Work out the finished part from the listing and answer in its coordinate system (mm). Face numbers are marked on the shaded views. A direction names the side the tool comes from. Round coordinates to 2 decimals unless told otherwise and drop trailing zeros. Order: outer loops, then holes, each group sorted by start corner. A loop starts at its lowest first (then second) coordinate and runs counter-clockwise, first axis right, second up. Notation, with made-up numbers: (-35, -21.5) - (23, -21.5) arc R14 cw to (23, -11.5) - close; hole circle Ø2 at (59, 7.5). An arc over 180 degrees is marked (long way). Answer in a Markdown table with one row per item.
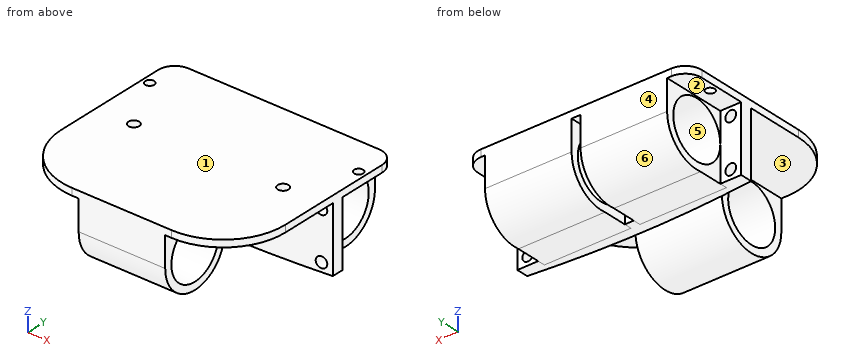
from build123d import *

# Parameters (mm, degrees)
SKETCH1_R            = 1.79994
SKETCH1_R_2          = 1.5
BOSS_EXTRUDE1_DEPTH  = 7
SKETCH2_W            = 75
SKETCH2_H            = 13.099999962
SKETCH2_R            = 2.6999438
SKETCH2_R_2          = 2.499995
SKETCH2_R_3          = 1.3498449
BOSS_EXTRUDE2_DEPTH  = 6.987999994
SKETCH2_3_R          = 2.6999438
SKETCH2_3_R_2        = 1.3498449
CUT_EXTRUDE1_DEPTH   = 2.5
SKETCH5_W            = 75
SKETCH5_H            = 13.099999962
CUT_EXTRUDE3_DEPTH   = 21.082
SKETCH6_W            = 75
SKETCH6_H            = 7
BOSS_EXTRUDE3_DEPTH  = 9.5
SKETCH8_W            = 75
SKETCH8_H            = 38.030205227
CUT_EXTRUDE4_DEPTH   = 4.666
SKETCH10_W           = 75
SKETCH10_H           = 2.334
BOSS_EXTRUDE5_DEPTH  = 35
SKETCH11_R           = 1.79994
CUT_EXTRUDE5_DEPTH   = 5
SKETCH15_W           = 44.653530321
SKETCH15_H           = 13.617301916
SKETCH15_W_2         = 11.728266088
SKETCH15_H_2         = 5.987537529
BOSS_EXTRUDE7_DEPTH  = 2.334
SKETCH16_R           = 9.5
BOSS_EXTRUDE9_DEPTH  = 29
SKETCH17_R           = 9.5
BOSS_EXTRUDE11_DEPTH = 14.5
FILLET5_R            = 20.828
FILLET6_R            = 5.588
BOSS_EXTRUDE13_DEPTH = 21.905881
CUT_EXTRUDE6_REACH   = 46
SKETCH21_R           = 1.8


with BuildPart() as part:
    # Sketch1 → Boss-Extrude1 (new body)
    with BuildSketch(Plane.XY):
        with BuildLine():
            Line((37.5, -10.5), (30, -10.5))
            ThreePointArc((30, -10.5), (25, -15.5), (20, -10.5))
            Line((20, -10.5), (5, -10.5))
            ThreePointArc((5, -10.5), (0, -15.5), (-5, -10.5))
            Line((-5, -10.5), (-20, -10.5))
            ThreePointArc((-20, -10.5), (-25, -15.5), (-30, -10.5))
            Line((-30, -10.5), (-37.5, -10.5))
            Line((-37.5, -10.5), (-37.5, 10.5))
            Line((-37.5, 10.5), (37.5, 10.5))
            Line((37.5, 10.5), (37.5, -10.5))
        make_face()
        with Locations((-25, -10.5)):
            Circle(SKETCH1_R, mode=Mode.SUBTRACT)
        with Locations((0, -10.5)):
            Circle(SKETCH1_R, mode=Mode.SUBTRACT)
        with Locations((25, -10.5)):
            Circle(SKETCH1_R, mode=Mode.SUBTRACT)
        with Locations((-35, 8)):
            Circle(SKETCH1_R_2, mode=Mode.SUBTRACT)
        with Locations((-15, 8)):
            Circle(SKETCH1_R_2, mode=Mode.SUBTRACT)
        with Locations((-10, 8)):
            Circle(SKETCH1_R_2, mode=Mode.SUBTRACT)
        with Locations((10, 8)):
            Circle(SKETCH1_R_2, mode=Mode.SUBTRACT)
        with Locations((35, 8)):
            Circle(SKETCH1_R_2, mode=Mode.SUBTRACT)
        with Locations((15, 8)):
            Circle(SKETCH1_R_2, mode=Mode.SUBTRACT)
    extrude(amount=BOSS_EXTRUDE1_DEPTH)

    # Sketch2 → Boss-Extrude2 (add)
    with BuildSketch(Plane(origin=(0, 2.24999999, 0), x_dir=(1, 0, 0), z_dir=(0, 1, 0))):
        with Locations((0, -13.549999981)):
            Rectangle(SKETCH2_W, SKETCH2_H)
        with Locations((31.0001404, -13.549999981)):
            Circle(SKETCH2_R, mode=Mode.SUBTRACT)
        with Locations((-31.0001404, -13.549999981)):
            Circle(SKETCH2_R, mode=Mode.SUBTRACT)
        with Locations((-25, -13.549999981)):
            Circle(SKETCH2_R_2, mode=Mode.SUBTRACT)
        with Locations((-6.0001404, -13.549999981)):
            Circle(SKETCH2_R, mode=Mode.SUBTRACT)
        with Locations((6.0001404, -13.549999981)):
            Circle(SKETCH2_R, mode=Mode.SUBTRACT)
        with Locations((0, -13.549999981)):
            Circle(SKETCH2_R_2, mode=Mode.SUBTRACT)
        with Locations((-18.9998596, -13.549999981)):
            Circle(SKETCH2_R, mode=Mode.SUBTRACT)
        with Locations((25, -13.549999981)):
            Circle(SKETCH2_R_2, mode=Mode.SUBTRACT)
        with Locations((18.9998596, -13.549999981)):
            Circle(SKETCH2_R, mode=Mode.SUBTRACT)
        with Locations((-31.0001404, -13.549999981)):
            Circle(SKETCH2_R)
        with Locations((-31.0001404, -13.549999981)):
            Circle(SKETCH2_R_3, mode=Mode.SUBTRACT)
        with Locations((-18.9998596, -13.549999981)):
            Circle(SKETCH2_R)
        with Locations((-18.9998596, -13.549999981)):
            Circle(SKETCH2_R_3, mode=Mode.SUBTRACT)
        with Locations((-6.0001404, -13.549999981)):
            Circle(SKETCH2_R)
        with Locations((-6.0001404, -13.549999981)):
            Circle(SKETCH2_R_3, mode=Mode.SUBTRACT)
        with Locations((6.0001404, -13.549999981)):
            Circle(SKETCH2_R)
        with Locations((6.0001404, -13.549999981)):
            Circle(SKETCH2_R_3, mode=Mode.SUBTRACT)
        with Locations((18.9998596, -13.549999981)):
            Circle(SKETCH2_R)
        with Locations((18.9998596, -13.549999981)):
            Circle(SKETCH2_R_3, mode=Mode.SUBTRACT)
        with Locations((31.0001404, -13.549999981)):
            Circle(SKETCH2_R)
        with Locations((31.0001404, -13.549999981)):
            Circle(SKETCH2_R_3, mode=Mode.SUBTRACT)
    extrude(amount=-BOSS_EXTRUDE2_DEPTH)

    # Sketch2<3> → Cut-Extrude1 (cut)
    with BuildSketch(Plane(origin=(0, 2.24999999, 0), x_dir=(1, 0, 0), z_dir=(0, 1, 0))):
        with Locations((-31.0001404, -13.549999981)):
            Circle(SKETCH2_3_R)
        with Locations((-31.0001404, -13.549999981)):
            Circle(SKETCH2_3_R_2, mode=Mode.SUBTRACT)
        with Locations((-18.9998596, -13.549999981)):
            Circle(SKETCH2_3_R)
        with Locations((-18.9998596, -13.549999981)):
            Circle(SKETCH2_3_R_2, mode=Mode.SUBTRACT)
        with Locations((-6.0001404, -13.549999981)):
            Circle(SKETCH2_3_R)
        with Locations((-6.0001404, -13.549999981)):
            Circle(SKETCH2_3_R_2, mode=Mode.SUBTRACT)
        with Locations((6.0001404, -13.549999981)):
            Circle(SKETCH2_3_R)
        with Locations((6.0001404, -13.549999981)):
            Circle(SKETCH2_3_R_2, mode=Mode.SUBTRACT)
        with Locations((18.9998596, -13.549999981)):
            Circle(SKETCH2_3_R)
        with Locations((18.9998596, -13.549999981)):
            Circle(SKETCH2_3_R_2, mode=Mode.SUBTRACT)
        with Locations((31.0001404, -13.549999981)):
            Circle(SKETCH2_3_R)
        with Locations((31.0001404, -13.549999981)):
            Circle(SKETCH2_3_R_2, mode=Mode.SUBTRACT)
    extrude(amount=-CUT_EXTRUDE1_DEPTH, mode=Mode.SUBTRACT)

    # Sketch5 → Cut-Extrude3 (cut)
    with BuildSketch(Plane(origin=(0, 2.24999999, 0), x_dir=(1, 0, 0), z_dir=(0, 1, 0))):
        with Locations((0, -13.549999981)):
            Rectangle(SKETCH5_W, SKETCH5_H)
    extrude(amount=-CUT_EXTRUDE3_DEPTH, mode=Mode.SUBTRACT)

    # Sketch6 → Boss-Extrude3 (add)
    with BuildSketch(Plane(origin=(0, 10.5, 0), x_dir=(1, 0, 0), z_dir=(0, 1, 0))):
        with Locations((0, -3.5)):
            Rectangle(SKETCH6_W, SKETCH6_H)
    extrude(amount=BOSS_EXTRUDE3_DEPTH)

    # Sketch8 → Cut-Extrude4 (cut)
    with BuildSketch(Plane(origin=(0, 0, 0), x_dir=(-1, 0, 0), z_dir=(0, 0, -1))):
        with Locations((0, 0.984897387)):
            Rectangle(SKETCH8_W, SKETCH8_H)
    extrude(amount=-CUT_EXTRUDE4_DEPTH, mode=Mode.SUBTRACT)

    # Sketch10 → Boss-Extrude5 (add)
    with BuildSketch(Plane(origin=(0, -45.5, 0), x_dir=(-1, 0, 0), z_dir=(0, -1, 0))):
        with Locations((0, -5.833)):
            Rectangle(SKETCH10_W, SKETCH10_H)
    extrude(amount=-BOSS_EXTRUDE5_DEPTH)

    # Sketch11 → Cut-Extrude5 (cut)
    with BuildSketch(Plane(origin=(0, 0, 4.666), x_dir=(-1, 0, 0), z_dir=(0, 0, -1))):
        with Locations((-25, -10.5)):
            Circle(SKETCH11_R)
        with Locations((0, -10.5)):
            Circle(SKETCH11_R)
        with Locations((25, -10.5)):
            Circle(SKETCH11_R)
    extrude(amount=-CUT_EXTRUDE5_DEPTH, mode=Mode.SUBTRACT)

    # Sketch15 → Boss-Extrude7 (add)
    with BuildSketch(Plane.XY.offset(7)):
        with Locations((1.804442165, 8.803924913)):
            Rectangle(SKETCH15_W, SKETCH15_H)
        with Locations((-1.501191344, -11.287680254)):
            Rectangle(SKETCH15_W_2, SKETCH15_H_2)
    extrude(amount=-BOSS_EXTRUDE7_DEPTH)


with BuildPart() as body_2:
    # Sketch16 → Boss-Extrude9 (new body)
    with BuildSketch(Plane(origin=(30.50000003, 0, 0), x_dir=(0, 0, -1), z_dir=(1, 0, 0))):
        with BuildLine():
            Line((-4.666, -4), (5.334, -4))
            Line((5.334, -4), (17.2398809, -4))
            Line((17.2398809, -4), (17.2398809, 6.5))
            ThreePointArc((17.2398809, 6.5), (14.334, 15.937253933), (5.334, 20))
            Line((5.334, 20), (-4.666, 20))
            Line((-4.666, 20), (-4.666, -4))
        make_face()
        with Locations((5.334, 8)):
            Circle(SKETCH16_R, mode=Mode.SUBTRACT)
    extrude(amount=-BOSS_EXTRUDE9_DEPTH)


with BuildPart() as body_3:
    # Mirror1: mirrored copy
    add(body_2.part.mirror(Plane(origin=(0, 0, 0), x_dir=(0, 0, 1), z_dir=(1, 0, 0))))

    # Combine1: union body 2, part
    add(body_2.part)
    add(part.part)

    # Sketch17 → Boss-Extrude11 (add, symmetric)
    with BuildSketch(Plane(origin=(0, 0, 0), x_dir=(0, 0, -1), z_dir=(1, 0, 0))):
        with BuildLine():
            Line((5.334, -45.5), (-4.666, -45.5))
            Line((-4.666, -45.5), (-4.666, -21.5))
            Line((-4.666, -21.5), (5.334, -21.5))
            ThreePointArc((5.334, -21.5), (17.334, -33.5), (5.334, -45.5))
        make_face()
        with Locations((5.334, -33.5)):
            Circle(SKETCH17_R, mode=Mode.SUBTRACT)
    extrude(amount=BOSS_EXTRUDE11_DEPTH, both=True)

    # Fillet5
    fillet5_edges = [body_3.edges().sort_by_distance(p)[0] for p in [
        (37.5, -45.5, 5.833),
        (-37.5, -45.5, 5.833),
    ]]
    fillet(fillet5_edges, radius=FILLET5_R)

    # Fillet6
    fillet6_edges = [body_3.edges().sort_by_distance(p)[0] for p in [
        (-37.5, 20, 5.833),
        (37.5, 20, 5.833),
    ]]
    fillet(fillet6_edges, radius=FILLET6_R)

    # Sketch20 → Boss-Extrude13 (add)
    with BuildSketch(Plane(origin=(0, 0, 4.666), x_dir=(-1, 0, 0), z_dir=(0, 0, -1))):
        with BuildLine():
            Line((-37.5, -1.5), (37.5, -1.5))
            Line((37.5, -1.5), (37.5, -5.5))
            ThreePointArc((37.5, -5.5), (0, -7.5), (-37.5, -5.5))
            Line((-37.5, -5.5), (-37.5, -1.5))
        make_face()
    extrude(amount=BOSS_EXTRUDE13_DEPTH)

    # Sketch21 → Cut-Extrude6 (cut, up to next)
    with BuildSketch(Plane(origin=(0, -1.5, 0), x_dir=(1, 0, 0), z_dir=(0, 1, 0)), mode=Mode.PRIVATE) as cut_extrude6_sk1:
        with Locations((34, 14.2398809)):
            Circle(SKETCH21_R)
    cut_extrude6_tool1 = extrude(cut_extrude6_sk1.sketch, amount=-CUT_EXTRUDE6_REACH, mode=Mode.PRIVATE) & body_3.part
    add(cut_extrude6_tool1.solids().sort_by_distance((34, -1.5, -14.239881))[0], mode=Mode.SUBTRACT)
    # Sketch21 → Cut-Extrude6 (cut, up to next)
    with BuildSketch(Plane(origin=(0, -1.5, 0), x_dir=(1, 0, 0), z_dir=(0, 1, 0)), mode=Mode.PRIVATE) as cut_extrude6_sk2:
        with Locations((34, -1.7601191)):
            Circle(SKETCH21_R)
    cut_extrude6_tool2 = extrude(cut_extrude6_sk2.sketch, amount=-CUT_EXTRUDE6_REACH, mode=Mode.PRIVATE) & body_3.part
    add(cut_extrude6_tool2.solids().sort_by_distance((34, -1.5, 1.760119))[0], mode=Mode.SUBTRACT)
    # Sketch21 → Cut-Extrude6 (cut, up to next)
    with BuildSketch(Plane(origin=(0, -1.5, 0), x_dir=(1, 0, 0), z_dir=(0, 1, 0)), mode=Mode.PRIVATE) as cut_extrude6_sk3:
        with Locations((-34, -1.7601191)):
            Circle(SKETCH21_R)
    cut_extrude6_tool3 = extrude(cut_extrude6_sk3.sketch, amount=-CUT_EXTRUDE6_REACH, mode=Mode.PRIVATE) & body_3.part
    add(cut_extrude6_tool3.solids().sort_by_distance((-34, -1.5, 1.760119))[0], mode=Mode.SUBTRACT)
    # Sketch21 → Cut-Extrude6 (cut, up to next)
    with BuildSketch(Plane(origin=(0, -1.5, 0), x_dir=(1, 0, 0), z_dir=(0, 1, 0)), mode=Mode.PRIVATE) as cut_extrude6_sk4:
        with Locations((-34, 14.2398809)):
            Circle(SKETCH21_R)
    cut_extrude6_tool4 = extrude(cut_extrude6_sk4.sketch, amount=-CUT_EXTRUDE6_REACH, mode=Mode.PRIVATE) & body_3.part
    add(cut_extrude6_tool4.solids().sort_by_distance((-34, -1.5, -14.239881))[0], mode=Mode.SUBTRACT)


solid = body_3.part
1) Find the intervals of material crossed by probe 1 along Z at (x, y) = (-34, -3.25); probe 2 along X at (y, z) = (-10.5, 6.1); probe 3 along X at (y, z) = (8, 5.7), in increasing order. Write a range as from..to.
Filled in:
| item | result |
|---|---|
| probe 1 | z = -17.24..-16.04, -12.44..-0.04, 3.56..7 |
| probe 2 | x = -37.5..-26.8, -23.2..23.2, 26.8..37.5 |
| probe 3 | x = -37.5..-36.5, -33.5..33.5, 36.5..37.5 |
2) The mould has two halves that part along Z. Classify the marked faces 4, 5 and 6: released by +Z, released by -Z, zero draft, split by the parting line, or undercut.
Filled in:
| item | result |
|---|---|
| face 4 | zero draft |
| face 5 | undercut |
| face 6 | released by -Z |
3) Find section C-C, the plane z = -8.75. Give the vertices of the cut face in (x, y) (1 decimal).
Filled in:
| item | result |
|---|---|
| outline | (-37.5, -5.5) arc R352.6 ccw to (37.5, -5.5) - (37.5, -1.5) - (30.5, -1.5) - (30.5, -0.9) - (1.5, -0.9) - (1.5, -1.5) - (-1.5, -1.5) - (-1.5, -0.9) - (-30.5, -0.9) - (-30.5, -1.5) - (-37.5, -1.5) - close; (-30.5, 16.9) - (-1.5, 16.9) - (-1.5, 19.5) - (-30.5, 19.5) - close; (-14.5, -45) - (14.5, -45) - (14.5, -42.4) - (-14.5, -42.4) - close; (-14.5, -24.6) - (14.5, -24.6) - (14.5, -22) - (-14.5, -22) - close; (1.5, 16.9) - (30.5, 16.9) - (30.5, 19.5) - (1.5, 19.5) - close |
4) Find section A-A, the plane y = 8. Give the vertices of the cut face in (x, z), then the cut area to 3 significant figures.
Filled in:
| item | result |
|---|---|
| outline | (-37.5, 4.67) - (-36.5, 4.67) - (-36.5, 7) - (-37.5, 7) - close; (-33.5, 4.67) - (-30.5, 4.67) - (-30.5, 4.17) - (-1.5, 4.17) - (-1.5, 4.67) - (1.5, 4.67) - (1.5, 4.17) - (30.5, 4.17) - (30.5, 4.67) - (33.5, 4.67) - (33.5, 7) - (-33.5, 7) - close; (-30.5, -17.33) - (-1.5, -17.33) - (-1.5, -14.83) - (-30.5, -14.83) - close; (1.5, -17.33) - (30.5, -17.33) - (30.5, -14.83) - (1.5, -14.83) - close; (36.5, 4.67) - (37.5, 4.67) - (37.5, 7) - (36.5, 7) - close |
| area | 335 mm^2 |
5) Which of the six approach directions +Z, -Z, +X, -X, +Y, -Y give full straight-line access (tool end or side, diameter ignored) to the marked faces 1, 2 and 3?
Filled in:
| item | result |
|---|---|
| face 1 | +Z, +X, -X, +Y, -Y |
| face 2 | -Z, -X, +Y |
| face 3 | -Z |
6) Each of these flat-tipped pins is pushed along its axis until it touches: pin 1 (4.5 mm diameter, centred on x = 25, y = -10.5, fed in from +Z); pin 2 (8.5 mm diameter, centred on x = -15, y = -0.5, fed in from -Z); pin 3 (11 mm diameter, centred on y = 5, z = -9.5, fed in from -X); pin 4 (12 mm diameter, centred on y = -29, z = -14, fed in from +X). Where does it stop, or does it pass through?
Filled in:
| item | result |
|---|---|
| pin 1 | stops at z = 7 |
| pin 2 | stops at z = -17.24 |
| pin 3 | stops at x = -30.5 |
| pin 4 | stops at x = 14.5 |
7) Find section D-D, the plane y = -33.5. Give the vertices of the cut face in (x, z).
Filled in:
| item | result |
|---|---|
| outline | (-35.54, 4.67) - (-14.5, 4.67) - (-14.5, 4.17) - (14.5, 4.17) - (14.5, 4.67) - (35.54, 4.67) - (35.54, 7) - (-35.54, 7) - close; (-14.5, -17.33) - (14.5, -17.33) - (14.5, -14.83) - (-14.5, -14.83) - close |
8) Find section B-B, the plane x = -25. Give the vertices of the cut face in (y, z).
Filled in:
| item | result |
|---|---|
| outline | (-43.76, 4.67) - (-12.3, 4.67) - (-12.3, 7) - (-43.76, 7) - close; (-8.7, 4.67) - (-6.61, 4.67) - (-6.61, -17.24) - (6.5, -17.24) arc R12 ccw to (20, -5.33) - (20, 7) - (-8.7, 7) - close; hole circle Ø19 at (8, -5.33) |
